Build history of the part. All positions in model axes, mm. Face numbers are marked on the shaded views. A direction names the side the tool comes from. Round coordinates to 2 decimals unless told otherwise and drop trailing zeros. Write each loop counter-clockwise with the first axis right and the second up, starting at its lowest first coordinate (ties: lowest second). Pieces come first, ordered by that corner, then holes. Notation, with made-up numbers: (45.25, -36) -> (99.25, -36) arc R18 cw to (99.25, -28) -> close; hole circle Ø3 at (4, -18). An arc over 180 degrees is marked (long way). Answer in a Markdown table with one row per item.
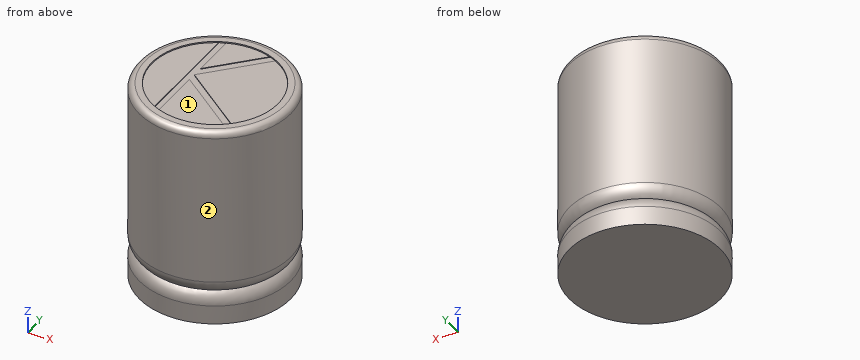
Autodesk Inventor part; units mm, degrees
ref_plane "Work Plane1" through (10, 0, 0) normal (1, 0, 0) x (0, 1, 0)
ref_plane "YZ Plane" through (0, 0, 0) normal (1, 0, 0) x (0, 1, 0)
ref_plane "XZ Plane" through (0, 0, 0) normal (0, 1, 0) x (-1, 0, 0)
sketch "Sketch1" plane through (0, 0, 0) normal (0, 0, 1) x (1, 0, 0)
  line L0 (0, 9.6) -> (0, -7.2) construction
  line L1 (-7.2, 0) -> (9.6, 0) construction
  circle A0 centre (0, 0) radius 6
  dimension "d0" = 12
extrude "Extrusion1" add sketch "Sketch1" along normal blind 16
sketch "Sketch6" plane through (0, 0, 0) normal (1, 0, 0) x (0, 1, 0)
  line L0 (0, 20.8) -> (0, -1.6)
  line L1 (6, 0) -> (6, 16)
  line L2 (6, 3.5) -> (6, 1.5)
  line L3 (6, 2.5) -> (5.5, 2.5) construction
  line L4 (-6, 0) -> (6, 0) construction
  arc A0 (5.5, 2.5) -> (6, 3.5) centre (4.75, 3.5) ccw
  arc A1 (6, 1.5) -> (5.5, 2.5) centre (4.75, 1.5) ccw
  point P0 (0, 0)
  dimension "d16" = 2
  dimension "d17" = 2.5
  dimension "d18" = 0.5
revolve "Revolution1" cut sketch "Sketch6" angle 360 about axis through (0, 0, 0) along (0, 0, -1)
sketch "Sketch2" plane through (0, 0, 16) normal (0, 0, 1) x (1, 0, 0)
  circle A0 centre (0, 0) radius 6
  circle A1 centre (0, 0) radius 5
  dimension "d3" = 1
extrude "Extrusion2" cut sketch "Sketch2" against normal blind 0.1 contours A1
sketch "Sketch3" plane through (0, 0, 15.9) normal (0, 0, 1) x (1, 0, 0)
  line L0 (-2.2779, 4.6629) -> (-1.8048, 4.6629)
  line L1 (-1.8048, 4.6629) -> (-1.8048, -4.9424)
  line L2 (-1.8048, -4.9424) -> (-2.2779, -4.9424)
  line L3 (-2.2779, -4.9424) -> (-2.2779, 4.6629)
  line L4 (-1.8048, 0.2777) -> (-2.233, 0.6841)
  line L5 (-2.233, 0.6841) -> (1.932, 5.0712)
  line L6 (1.932, 5.0712) -> (2.3602, 4.6648)
  line L7 (2.3602, 4.6648) -> (-1.8048, 0.2777)
  line L8 (-1.8048, 0.2777) -> (-2.1189, -0.1414)
  line L9 (-2.1189, -0.1414) -> (3.111, -4.0616)
  line L10 (3.111, -4.0616) -> (3.4251, -3.6426)
  line L11 (3.4251, -3.6426) -> (-1.8048, 0.2777)
  circle A0 centre (0, 0) radius 5
extrude "Extrusion3" cut sketch "Sketch3" against normal blind 0.05 contours L0 A0 L3 | L1 L5 L4 L8 L9 A0 L3 | L5 A0 L7 L1 | L1 L4 L5 | L5 L6 L7 A0 | A0 L1 L2 L3 | L11 A0 L9 L1 | L1 L9 L8 | L10 L9 A0
fillet "Fillet1" radius 0.5 1 edges at (-6, 0, 16)
sketch "Sketch5" plane through (0, 0, 16) normal (0, 0, 1) x (1, 0, 0)
  circle A0 centre (0, 0) radius 5
  circle A1 centre (0, 0) radius 6
  line L0 (2, -4.5826) -> (2, -7)
  line L1 (2, -7) -> (-2, -7)
  line L2 (-2, -7) -> (-2, -4.5826)
  line L3 (0, -7.2) -> (0, 9.6)
  point P0 (0, -6)
  point P1 (0, -6)
  dimension "d12" = 1
  dimension "d13" = 4
split_face "Split1"
ref_plane "Work Plane1" through (10, 0, 0) normal (1, 0, 0) x (0, 1, 0)
properties part number "config - capasitor 3500 μF"
Q1. Saw through at B-B on z = 3. Write the cut outline in (x, y).
A:
| item | result |
|---|---|
| outline | circle Ø11.79 at (0, 0) |
Q2. Which spindle directions (+Z, -Z, +X, -X, +Y, -Y) get a long thin tool onto all of the face, cutting with end or side? Do the marked faces 1 and 2. Say none if no direction does.
A:
| item | result |
|---|---|
| face 1 | +Z |
| face 2 | +Z, -Z |
Q3. Wall check: line 1 (Z direction, x = -4.25, y = -1); line 2 (Y direction, x = -3.75, z = 13.75); line 3 (Y direction, x = -1, z = 9). Give the ranges that are in metal, low to high. Write a range as [from, to].
A:
| item | result |
|---|---|
| line 1 | [0, 15.9] |
| line 2 | [-4.68, 4.68] |
| line 3 | [-5.92, 5.92] |
Q4. Saw through at A-A on z = 13.25. Write the cut outline in (x, y).
A:
| item | result |
|---|---|
| outline | circle Ø12 at (0, 0) |
Q5. Drop flat-ended pins along their axis: P1, Ø3, axis at y = -2.5, z = 8.5, coming from the +X side; P2, Ø4, axis at x = -2.5, y = -1, coming from the +Z side; P3, Ø1.5, axis at y = 3, z = 11, coming from the -X side. Give the stop position or say it passes through.
A:
| item | result |
|---|---|
| P1 | x = 5.92 |
| P2 | z = 15.9 |
| P3 | x = -5.56 |
